Work out the finished part from the listing and answer in its coordinate system (mm). A direction names the side the tool comes from. Coordinates: 2 decimals unless noted, no trailing zeros. Order: outer loops, then holes, each group sorted by start corner. A loop starts at its lowest first (then second) coordinate and runs counter-clockwise, first axis right, second up.
1. The part is cut by section A-A, the plane z = 6. Give the vertices of the cut face in (x, y).
2. The part is cut by section D-D, the plane z = -12.5. Give the vertices of the cut face in (x, y), then the cut area to 3 significant figures.
3. The part is cut by section C-C, the plane x = -36.5. Give the vertices of the cut face in (y, z), then the cut area to 3 significant figures.
4. The part is cut by section B-B, the plane y = 36.5. Give the vertices of the cut face in (x, z), then the cut area to 3 significant figures.
5. A tool of negligible diameter and unlimited length cuts with its end or side. For faces 1 (the cylindrical face through (-35.3, 35.6, 3.9)), 2 (the flat face through (-21, 0, 24)), from which of +Z, -Z, +X, -X, +Y, -Y can it reach the whole face along a straight path? Write none if from no direction.
6. Find the intervals of material crossed by probe 1 along X at (y, z) = (36, 4); probe 2 along Z at (x, y) = (-2, 39); probe 3 along Z at (x, y) = (-30.5, 22.5), in increasing order.
7. Determine the mould class of faces 3 (the flat face through (-36, 6, 8)), 4 (the flat face through (-21, 21, -25)), 5 (the cylindrical face through (-19.16, 22.69, -13.34)) for opening direction X: +X half, -X half, draft (parallel to the pull), parting line (faces both ways), or undercut.
8. Flat-ended cylindrical pins translate along their axes: pin 1 Ø2 at (x, z) = (-21, 26.5) entering from -Y; pin 2 Ø1.8 at (x, y) = (-5.5, 36.5) entering from -Z; pin 3 Ø4 at (x, y) = (-36.5, 36.5) entering from -Z; pin 4 Ø12.5 at (x, y) = (-30.5, 31) entering from -Z. Find the tip coordinate at first contact, or state that the pin passes through.
```python
from build123d import *

# Parameters (mm, degrees)
SKETCH_1_W          = 42
SKETCH_1_H          = 42
EXTRUDE_1_DEPTH     = 48
SKETCH_3_R          = 11
EXTRUDE_2_DEPTH     = 2
SKETCH_4_R          = 2.5
EXTRUDE_3_DEPTH     = 23
SKETCH_5_R          = 1.5
CUT_EXTRUDE_1_DEPTH = 8


with BuildPart() as part:
    # 草图1 → 凸台-拉伸1 (new body)
    with BuildSketch(Plane.XY):
        with Locations((-21, 21)):
            Rectangle(SKETCH_1_W, SKETCH_1_H)
    extrude(amount=EXTRUDE_1_DEPTH)

    # 草图3 → 凸台-拉伸2 (add)
    with BuildSketch(Plane(origin=(0, 0, 0), x_dir=(-1, 0, 0), z_dir=(0, 0, -1))):
        with Locations((21, 21)):
            Circle(SKETCH_3_R)
    extrude(amount=EXTRUDE_2_DEPTH)

    # 草图4 → 凸台-拉伸3 (add)
    with BuildSketch(Plane(origin=(0, 0, -2), x_dir=(-1, 0, 0), z_dir=(0, 0, -1))):
        with Locations((21, 21)):
            Circle(SKETCH_4_R)
    extrude(amount=EXTRUDE_3_DEPTH)

    # 草图5 → 切除-拉伸1 (cut)
    with BuildSketch(Plane(origin=(0, 0, 0), x_dir=(-1, 0, 0), z_dir=(0, 0, -1))):
        with Locations((5.5, 5.5)):
            Circle(SKETCH_5_R)
        with Locations((36.5, 5.5)):
            Circle(SKETCH_5_R)
        with Locations((36.5, 36.5)):
            Circle(SKETCH_5_R)
        with Locations((5.5, 36.5)):
            Circle(SKETCH_5_R)
    extrude(amount=-CUT_EXTRUDE_1_DEPTH, mode=Mode.SUBTRACT)


solid = part.part
```
Geometry says:
1. outline: (-42, 0) - (0, 0) - (0, 42) - (-42, 42) - close; hole circle Ø3 at (-36.5, 5.5); hole circle Ø3 at (-36.5, 36.5); hole circle Ø3 at (-5.5, 5.5); hole circle Ø3 at (-5.5, 36.5)
2. outline: circle Ø5 at (-21, 21)
2. area: 19.6 mm2
3. outline: (0, 0) - (4, 0) - (4, 8) - (7, 8) - (7, 0) - (35, 0) - (35, 8) - (38, 8) - (38, 0) - (42, 0) - (42, 48) - (0, 48) - close
3. area: 1,970 mm2
4. outline: (-42, 0) - (-38, 0) - (-38, 8) - (-35, 8) - (-35, 0) - (-7, 0) - (-7, 8) - (-4, 8) - (-4, 0) - (0, 0) - (0, 48) - (-42, 48) - close
4. area: 1,970 mm2
5. face 1: -Z
5. face 2: +Z, -Z, +X, -X, -Y
6. probe 1: x = -42 to -37.91, -35.09 to -6.91, -4.09 to 0
6. probe 2: z = 0 to 48
6. probe 3: z = -2 to 48
7. face 3: undercut
7. face 4: draft
7. face 5: parting line
8. pin 1: stops at y = 0
8. pin 2: stops at z = 8
8. pin 3: stops at z = 0
8. pin 4: stops at z = -2
